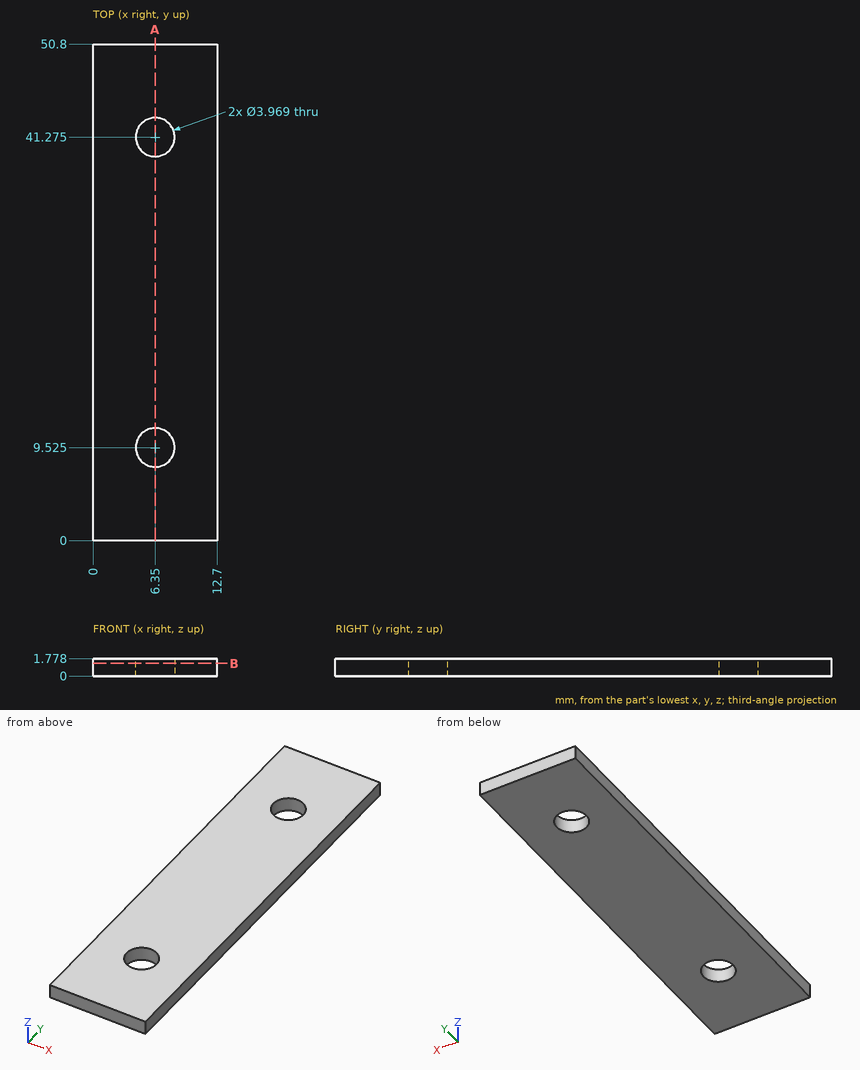
Check sheet for the drawn part. Datum: minimum x, y, z corner. Units: mm. Coordinates: 2 decimals unless noted, no trailing zeros. Loops run counter-clockwise (first coordinate to the right, second up) from the corner with the lowest first, then second, coordinate; pieces in that order, holes last. Notation, with made-up numbers: (78.5, -32.5) - (115.5, -32.5) arc R27 cw to (115.5, 3.5) - close; hole circle Ø2 at (18, -22.75). An arc over 180 degrees is marked (long way). Put each result on its own line as item: value.
Item 1: Section check A-A (x = 6.35). Enter the section's corners in (y, z), then the cut area to 3 significant figures.
Conclusion:
outline: (0, 0) - (7.54, 0) - (7.54, 1.78) - (0, 1.78) - close; (11.51, 0) - (39.29, 0) - (39.29, 1.78) - (11.51, 1.78) - close; (43.26, 0) - (50.8, 0) - (50.8, 1.78) - (43.26, 1.78) - close
area: 76.2 mm2
Item 2: Section check B-B (z = 1.3). Give the number of separate pieces and of enclosed holes in the cut face, then the cut area to 3 significant figures.
Conclusion:
separate pieces: 1
enclosed holes: 2
area: 620 mm2
Item 3: Scan lines: line 1 along Y through (x, z) = (6.35, 0.7); line 2 along Y through (x, z) = (6, 1.6); line 3 along X through (y, z) = (42, 1.4). Record each from-to range of solid material in increasing order.
Conclusion:
line 1: y = 0 to 7.54, 11.51 to 39.29, 43.26 to 50.8
line 2: y = 0 to 7.57, 11.48 to 39.32, 43.23 to 50.8
line 3: x = 0 to 4.5, 8.2 to 12.7
